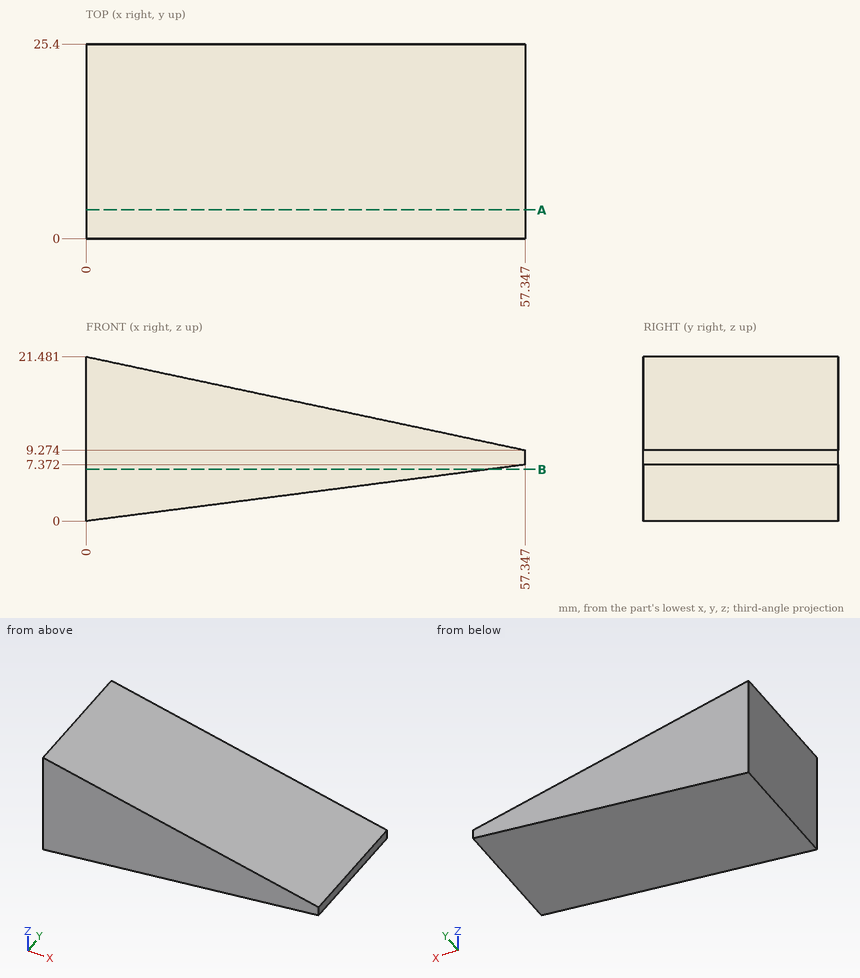
Can you work these out from the drawing? Everything is in mm from the part's minimum corner. Coordinates: 2 decimals unless noted, no trailing zeros. Write each loop counter-clockwise with the first axis right and the second up, starting at its lowest first coordinate (ties: lowest second). Pieces come first, ordered by that corner, then holes. Notation, with made-up numbers: (19.25, -17) -> (35.25, -17) arc R12 ccw to (35.25, -2) -> close; hole circle Ø4 at (-26, 13). An arc over 180 degrees is marked (long way). Write item = value, one per line.
(1) Imagine slicing it at B-B (z = 6.75). Please give me the cut outline in (x, y).
Verdict:
outline = (0, 0) -> (52.51, 0) -> (52.51, 25.4) -> (0, 25.4) -> close
(2) Imagine slicing it at A-A (y = 3.75). Please give me the cut outline in (x, z).
Verdict:
outline = (0, 0) -> (57.35, 7.37) -> (57.35, 9.27) -> (0, 21.48) -> close
(3) For pin 1 (10 mm diameter, centred on x = 20.5, y = 9, fed in from -Z); pin 2 (5 mm diameter, centred on x = 33.5, y = 13.5, fed in from -Z) (1 decimal); pin 3 (5 mm diameter, centred on x = 28.5, y = 7, fed in from -Z), each with a flat end and sliding along its axis, tell me the tip position at first contact or that it passes through.
Verdict:
pin_1 = 1.99
pin_2 = 4
pin_3 = 3.34
(4) If I drill on probe 1 along Z at (x, y) = (10, 9.25) (1 decimal); probe 2 along Z at (x, y) = (26.5, 17), over which ranges is the centre line in solid material (lowest first)?
Verdict:
probe_1 = 1.3 to 19.4
probe_2 = 3.41 to 15.84
